```python
from build123d import *

# Parameters (mm, degrees)
PAD_DEPTH            = 120
PAD001_DEPTH         = 80
POCKET_DEPTH         = 5.767281
POCKET_DEPTH_BACK    = 5.767281
POCKET001_DEPTH      = 25.767281
POCKET002_DEPTH      = 5.767281
POCKET002_DEPTH_BACK = 5.767281
POCKET003_DEPTH      = 5.767281
POCKET003_DEPTH_BACK = 5.767281
POCKET004_DEPTH      = 5.767281
POCKET004_DEPTH_BACK = 5.767281
FILLET_R             = 1


with BuildPart() as part:
    # Sketch → Pad (new body)
    with BuildSketch(Plane.XZ):
        with BuildLine():
            ThreePointArc((-4, -3), (0, -5), (4, -3))
            Line((4, -3), (5.766281, -3))
            ThreePointArc((-5.766281, -3), (0, -6.5), (5.766281, -3))
            Line((-4, -3), (-5.766281, -3))
        make_face()
    extrude(amount=PAD_DEPTH)

    # Sketch001 → Pad001 (join)
    with BuildSketch(Plane.XZ):
        with BuildLine():
            ThreePointArc((-3, -5.766281), (0, -6.5), (3, -5.766281))
            Line((3, -25.766281), (3, -5.766281))
            Line((-3, -25.766281), (3, -25.766281))
            Line((-3, -5.766281), (-3, -25.766281))
        make_face()
    extrude(amount=PAD001_DEPTH)

    # Sketch002 → Pocket (cut, two sides)
    with BuildSketch(Plane.YZ) as pocket_sk:
        Polygon((-30, -18), (-30, -6), (-90, -6), (-90, -10), (-35, -10), (-35, -18), align=None)
    extrude(amount=-POCKET_DEPTH, mode=Mode.SUBTRACT)
    extrude(pocket_sk.sketch, amount=POCKET_DEPTH_BACK, mode=Mode.SUBTRACT)

    # Sketch003 → Pocket001 (cut, through all)
    with BuildSketch(Plane.XY):
        with BuildLine():
            Line((-10, -104), (-10, -134))
            Line((-10, -134), (10, -134))
            Line((10, -134), (10, -104))
            Line((10, -104), (4, -112))
            ThreePointArc((-4, -112), (0, -114), (4, -112))
            Line((-4, -112), (-10, -104))
        make_face()
    extrude(amount=-POCKET001_DEPTH, mode=Mode.SUBTRACT)

    # Sketch004 → Pocket002 (cut, two sides)
    with BuildSketch(Plane.YZ) as pocket002_sk:
        Polygon((-43, -18), (-43, -6), (-103, -6), (-103, -10), (-48, -10), (-48, -18), align=None)
    extrude(amount=-POCKET002_DEPTH, mode=Mode.SUBTRACT)
    extrude(pocket002_sk.sketch, amount=POCKET002_DEPTH_BACK, mode=Mode.SUBTRACT)

    # Sketch005 → Pocket003 (cut, two sides)
    with BuildSketch(Plane.YZ) as pocket003_sk:
        Polygon((-56, -18), (-56, -6), (-116, -6), (-116, -10), (-61, -10), (-61, -18), align=None)
    extrude(amount=-POCKET003_DEPTH, mode=Mode.SUBTRACT)
    extrude(pocket003_sk.sketch, amount=POCKET003_DEPTH_BACK, mode=Mode.SUBTRACT)

    # Sketch006 → Pocket004 (cut, two sides)
    with BuildSketch(Plane.YZ) as pocket004_sk:
        Polygon((-69, -18), (-69, -6), (-129, -6), (-129, -10), (-74, -10), (-74, -18), align=None)
    extrude(amount=-POCKET004_DEPTH, mode=Mode.SUBTRACT)
    extrude(pocket004_sk.sketch, amount=POCKET004_DEPTH_BACK, mode=Mode.SUBTRACT)

    # Fillet
    fillet_edges = [part.edges().sort_by_distance(p)[0] for p in [
        (0, -74, -10),
        (-3, -77, -10),
        (0, -80, -10),
        (3, -77, -10),
        (0, -61, -10),
        (-3, -65, -10),
        (0, -69, -10),
        (3, -65, -10),
        (0, -48, -10),
        (-3, -52, -10),
        (0, -56, -10),
        (3, -52, -10),
        (0, -35, -10),
        (-3, -39, -10),
        (0, -43, -10),
        (3, -39, -10),
        (-3, -40, -25.766281),
        (3, -40, -25.766281),
        (0, 0, -25.766281),
        (0, -80, -25.766281),
    ]]
    fillet(fillet_edges, radius=FILLET_R)


solid = part.part
```
Input: part model. Units: mm. Frame: model coordinates. A direction names the side the tool comes from. Coordinates: 2 decimals unless noted, no trailing zeros. Write each loop counter-clockwise with the first axis right and the second up, starting at its lowest first coordinate (ties: lowest second). Pieces come first, ordered by that corner, then holes. Notation, with made-up numbers: M 41.5,73 L 61.5,73 A26 ccw 61.5,98 Z; hole C 61,73.25 d6. An arc over 180 degrees is marked long. Use one line per item in the form item = value.
Q1. Material intervals for probe 1 along Y at (x, z) = (0.25, -12.25); probe 2 along X at (y, z) = (-14, -12.5); probe 3 along Y at (x, z) = (-2, -22), sorted ascending. Write a range as from..to.
Answer below:
probe_1 = -80..-74, -69..-61, -56..-48, -43..-35, -30..0
probe_2 = -3..3
probe_3 = -80..0
Q2. First-contact query: pin 1 (1.5 mm diameter, centred on x = 1, y = -33.5, fed in from +Z); pin 2 (5.5 mm diameter, centred on x = -1.5, y = -46, fed in from +Z); pin 3 (3 mm diameter, centred on x = 1, z = -16, fed in from -Y); pin 4 (1 mm diameter, centred on y = -68.5, z = -21.5, fed in from -X). Flat tips, straight axial feed; report the tip coordinate or a pass-through.
Answer below:
pin_1 = -4.68
pin_2 = -3
pin_3 = -80
pin_4 = -3
Q3. Set-up query: faces 4 (the face through (0, -30, -12)), 5 (the face through (0, -80, -18)), 6 (the face through (0, -71, -6)), 7 (the face through (-3, -39, -17)). Return all of +Z, -Z, +X, -X, +Y, -Y with unobstructed straight access to the full face (end or side cutting, diameter ignored); none if empty.
Answer below:
face_4 = +X, -X
face_5 = -Z, +X, -X, -Y
face_6 = +X, -X, -Y
face_7 = -Z, -X, +Y, -Y
Q4. Section B-B (z = -12.75). Return loops of the section in (x, y).
Answer below:
outline = M -3,-80 L 3,-80 L 3,-74 L -3,-74 Z; M -3,-69 L 3,-69 L 3,-61 L -3,-61 Z; M -3,-56 L 3,-56 L 3,-48 L -3,-48 Z; M -3,-43 L 3,-43 L 3,-35 L -3,-35 Z; M -3,-30 L 3,-30 L 3,0 L -3,0 Z
Q5. Section C-C (y = -84). Return loops of the section in (x, z), plus the area to 3 significant figures.
Answer below:
outline = M -5.77,-3 A6.5 ccw -2.5,-6 L 2.5,-6 A6.5 ccw 5.77,-3 L 4,-3 A5 cw -4,-3 Z
area = 15.9 mm²
Q6. Section A-A (y = -57.5). Return loops of the section in (x, z), plus the area to 3 significant figures.
Answer below:
outline = M -5.77,-3 A6.5 ccw -3,-5.77 L -3,-6 L 3,-6 L 3,-5.77 A6.5 ccw 5.77,-3 L 4,-3 A5 cw -4,-3 Z; M -3,-24.77 A1 ccw -2,-25.77 L 2,-25.77 A1 ccw 3,-24.77 L 3,-18 L -3,-18 Z
area = 62.2 mm²
Q7. Draft query along Y for faces 1 (the face through (4.7, -111.07, -3.81)), 2 (the face through (5, -55, -3)), 3 (the face through (0, -69, -15)). Return one class per face: released by +Y, released by -Y, zero draft, split by the parting line, or undercut.
Answer below:
face_1 = released by -Y
face_2 = zero draft
face_3 = undercut
